from build123d import *

# Parameters (mm, degrees)
F0_W     = 834.7400754492
F0_H     = 50.8
F1_DEPTH = 3.048
F3_W     = 57.9247
F3_H     = 5.08
F3_W_2   = 115.8494
F4_DEPTH = 3.048
F6_DEPTH = 3.048
F7_DEPTH = 3.049
F8_W     = 6.096
F8_H     = 6.096
F8_R     = 2.8702
F8_R_2   = 4.953
F8_R_3   = 7.9375
F9_DEPTH = 3.049


# Not quite as in the source:
# - a feature names something its author has since deleted; it is built from what else it names


with BuildPart() as f1:
    # F0 (on Front) → F1 (new body)
    with BuildSketch(Plane.XZ):
        with Locations((417.3700377246, 25.4)):
            Rectangle(F0_W, F0_H)
    extrude(amount=F1_DEPTH)

    # F3 (on face) → F4 (join)
    with BuildSketch(Plane.XZ.offset(3.048)):
        with Locations((28.96235, 53.34)):
            Rectangle(F3_W, F3_H)
        with Locations((139.1233459082, 53.34)):
            Rectangle(F3_W_2, F3_H)
        with Locations((278.2466918164, 53.34)):
            Rectangle(F3_W_2, F3_H)
        with Locations((417.3700377246, 53.34)):
            Rectangle(F3_W_2, F3_H)
        with Locations((556.4933836328, 53.34)):
            Rectangle(F3_W_2, F3_H)
        with Locations((695.616729541, 53.34)):
            Rectangle(F3_W_2, F3_H)
        with Locations((805.7777254492, 53.34)):
            Rectangle(F3_W, F3_H)
    extrude(amount=-F4_DEPTH)

    # F5 (on face) → F6 (join)
    with BuildSketch(Plane.XZ.offset(3.048)):
        Polygon((-6.35, 6.35), (0, 6.35), (0, 44.45), (-6.35, 44.45), (-9.525, 47.625), (-9.525, 3.175), align=None)
    extrude(amount=-F6_DEPTH)

    # F5 (on face) → F7 (cut, through all)
    with BuildSketch(Plane.XZ.offset(3.048)):
        Polygon((828.3900754492, 8.89), (834.7400754492, 8.89), (834.7400754492, 46.99), (828.3900754492, 46.99), (825.2150754492, 50.165), (825.2150754492, 5.715), align=None)
    extrude(amount=-F7_DEPTH, mode=Mode.SUBTRACT)

    # F8 (on face) → F9 (cut, through all)
    with BuildSketch(Plane.XZ.offset(3.048)):
        with Locations((256.3264918164, 15.621)):
            Rectangle(F8_W, F8_H)
        with Locations((278.2466918164, 15.621)):
            Rectangle(F8_W, F8_H)
        with Locations((300.1668918164, 15.621)):
            Rectangle(F8_W, F8_H)
        with Locations((235.7016918164, 15.621)):
            Circle(F8_R)
        with Locations((323.9666918164, 15.621)):
            Circle(F8_R_2)
        with Locations((278.2466918164, 34.671)):
            Circle(F8_R_3)
    extrude(amount=-F9_DEPTH, mode=Mode.SUBTRACT)


solid = f1.part
The listing builds one solid part. Answer for the finished solid, in the listing's coordinates (mm). Round coordinates to 2 decimals unless told otherwise and drop trailing zeros. Write each question's results on one line, items separated by ' | '. Start each with the question number.
1) Find section A-A on y = -0.55. Count the separate pieces of the cut face and the enclosed holes in it, plus the area to 3 significant figures.
2) Each of these flat-tipped pins is pushed along its axis until it touches: pin 1 (0.9 mm diameter, centred on y = -2, z = 17, fed in from +X); pin 2 (0.9 mm diameter, centred on x = 67.5, y = -2, fed in from +Z). Where does it stop, or does it pass through?
3) Straight lines are drawn through the part: probe 1 along Z at (x, y) = (258, -2.15); probe 2 along X at (y, z) = (-1.15, 18) (1 decimal); probe 3 along X at (y, z) = (-2.15, 6) (3 decimals). For each, find the intervals that lie inside material, in ascending order.
Final values:
1) separate pieces: 1 | enclosed holes: 6 | area: 45,500 mm²
2) pin 1: x = 825.22 | pin 2: z = 50.8
3) probe 1: 0 to 12.57, 18.67 to 55.88 | probe 2: -9.5 to 234.1, 237.3 to 253.3, 259.4 to 275.2, 281.3 to 297.1, 303.2 to 319.6, 328.3 to 825.2 | probe 3: -9.525 to -6.7, 0 to 825.215, 825.5 to 834.74
